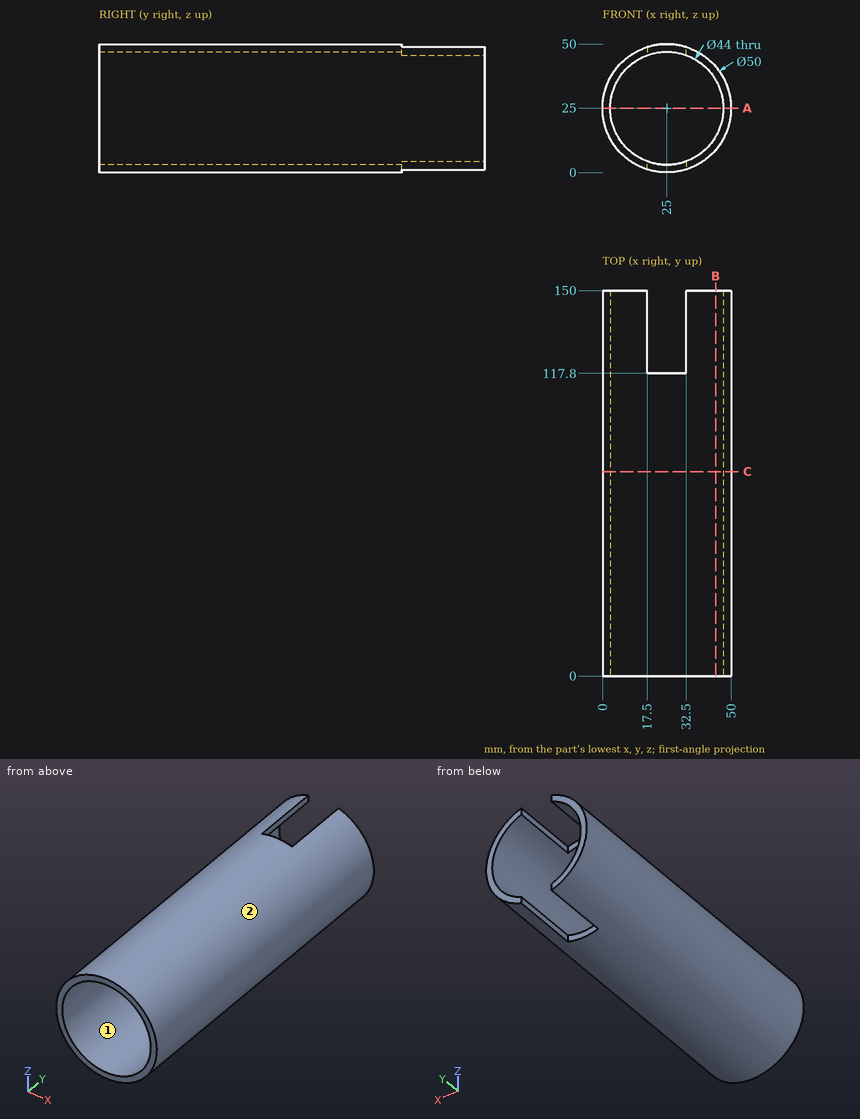
Drawing for the job (mm, zero at the part's lowest x, y, z). Round coordinates to 2 decimals unless told otherwise and drop trailing zeros. Write each loop counter-clockwise with the first axis right and the second up, starting at its lowest first coordinate (ties: lowest second). Pieces come first, ordered by that corner, then holes. Notation, with made-up numbers: M -37,3 L -7,3 A16 cw -7,28 Z; hole C 63,68 d5. An arc over 180 degrees is marked long. Put each result on its own line as item: value.
Item 1: Cut at A-A (z = 25). List the corners of the cut face in (x, y), and give its area (3 significant figures).
Responses:
outline: M 0,0 L 3,0 L 3,150 L 0,150 Z; M 47,0 L 50,0 L 50,150 L 47,150 Z
area: 900 mm²
Item 2: Cut at C-C (y = 79.5). List the corners of the cut face in (x, z), and give its area (3 significant figures).
Responses:
outline: C 25,25 d50; hole C 25,25 d44
area: 443 mm²
Item 3: Probe L1, parallel to Z at x = 25, y = 109; L2, parallel to Z at x = 19, y = 107.5. List the from-to ranges inside material, lowest first. Write a range as from..to.
Responses:
L1: 0..3, 47..50
L2: 0.73..3.83, 46.17..49.27
Item 4: Flat gauge pins, fed straight in: P1, Ø1.5, axis at x = 16.5, y = 91.5, coming from the +Z side; P2, Ø8, axis at y = 28.5, z = 44.5, coming from the +X side; P3, Ø3.5, axis at x = 27.5, z = 49, coming from the +Y side; P4, Ø2, axis at x = 18, z = 5, coming from the +Y side. Where does each tip first touch, or does it go through?
Responses:
P1: z = 48.77
P2: x = 44.62
P3: y = 117.8
P4: y = 150
Item 5: Mould opens along X. For the marked faces 1 and 2 say: +X half, -X half, draft (parallel to the pull), parting line (faces both ways), or undercut.
Responses:
face 1: undercut
face 2: parting line
Item 6: Cut at B-B (x = 44). List the corners of the cut face in (y, z), and give its area (3 significant figures).
Responses:
outline: M 0,8.75 L 150,8.75 L 150,13.91 L 0,13.91 Z; M 0,36.09 L 150,36.09 L 150,41.25 L 0,41.25 Z
area: 1,550 mm²
